The model under review builds one solid part; all positions refer to its coordinate system, in mm. A direction names the side the tool comes from. Give positions to 0.01 mm unless a question says otherwise; leave off trailing zeros. Order: outer loops, then holes, each group sorted by start corner. A loop starts at its lowest first (then second) coordinate and runs counter-clockwise, first axis right, second up. Notation, with made-up numbers: (30, 52) -> (63, 52) arc R34 cw to (63, 90) -> close; hole circle Ø8 at (81.25, -4.75). An arc over 180 degrees is marked (long way). Use one line per item in the form item = value.
Autodesk Inventor part; units mm, degrees
ref_plane "YZ Plane" through (0, 0, 0) normal (1, 0, 0) x (0, 1, 0)
ref_plane "XZ Plane" through (0, 0, 0) normal (0, 1, 0) x (-1, 0, 0)
ref_plane "XY Plane" through (0, 0, 0) normal (0, 0, 1) x (1, 0, 0)
sketch "Esboço1" plane through (0, 0, 0) normal (0, 0, 1) x (1, 0, 0)
  circle A0 centre (0, 0) radius 3
  dimension "d0" = 6
extrude "Extrusão1" add sketch "Esboço1" along normal mid plane 16
sketch "Esboço2" plane through (0, 0, 0) normal (1, 0, 0) x (0, 1, 0)
  line L0 (3.25, -6) -> (2.5, -6)
  line L1 (2.5, -6) -> (2.5, -6.75)
  line L2 (2.5, -6.75) -> (3.25, -6.75)
  line L3 (3.25, -6.75) -> (3.25, -6)
  line L4 (3.1313, 6.75) -> (2.5, 6.75)
  line L5 (2.5, 6.75) -> (2.5, 6)
  line L6 (2.5, 6) -> (3.1313, 6)
  line L7 (3.1313, 6) -> (3.1313, 6.75)
  line L8 (0, 0) -> (0, -8)
  line L9 (-3, -8) -> (3, -8)
  dimension "d3" = 5
  dimension "d4" = 6.5
  dimension "d5" = 6
  dimension "d6" = 0.75
  dimension "d7" = 6
  dimension "d8" = 0.75
revolve "Revolução1" cut sketch "Esboço2" angle 360 about axis through (0, 0, 0) along (0, 0, -1)
chamfer "Chanfro1" distance 0.3 angle 45 2 edges at (-3, 0, 8) (-3, 0, -8)
1. Add section A-A on y = 0. Give the boundary of the cut face in (x, z), then the cut area to 3 significant figures.
Values:
outline = (-3, -7.7) -> (-2.7, -8) -> (2.7, -8) -> (3, -7.7) -> (3, -6.75) -> (2.5, -6.75) -> (2.5, -6) -> (3, -6) -> (3, 6) -> (2.5, 6) -> (2.5, 6.75) -> (3, 6.75) -> (3, 7.7) -> (2.7, 8) -> (-2.7, 8) -> (-3, 7.7) -> (-3, 6.75) -> (-2.5, 6.75) -> (-2.5, 6) -> (-3, 6) -> (-3, -6) -> (-2.5, -6) -> (-2.5, -6.75) -> (-3, -6.75) -> close
area = 94.3 mm^2
2. The part is to be moulded in two halves that separate along Z. For faces 3 (the face through (2, -2, 6)), 4 (the face through (0, 0, -8)), 5 (the face through (0, 0, 8)), say which applies: +Z half, -Z half, draft (parallel to the pull), parting line (faces both ways), or undercut.
Values:
face_3 = undercut
face_4 = -Z half
face_5 = +Z half
3. Tool access review of faces 1 (the face through (-3, 0, 0)), 2 (the face through (2, -2, 6.75)): name each direction out of +Z, -Z, +X, -X, +Y, -Y from which nothing blocks a thin tool from reaching the whole face with its end or side.
Values:
face_1 = +Z, -Z
face_2 = none
4. Add section C-C on z = -3.75. Give the boundary of the cut face in (x, y), then the cut area to 3 significant figures.
Values:
outline = circle Ø6 at (0, 0)
area = 28.3 mm^2
5. For L1, parallel to Z at x = 0.55, y = 2.5; L2, parallel to Z at x = 1.85, y = 2.05; L3, parallel to X at y = -2.6, z = -0.5, list the stretches that pass through material, from the lowest coordinate up.
Values:
L1 = -8 to -6.75, -6 to 6, 6.75 to 8
L2 = -7.94 to -6.75, -6 to 6, 6.75 to 7.94
L3 = -1.5 to 1.5
6. For pin 1 Ø1.5 at (x, z) = (1.5, 5.5) entering from +Y, flat-tipped, find the tip position at first contact; note if it passes through.
Values:
pin_1 = 2.9
